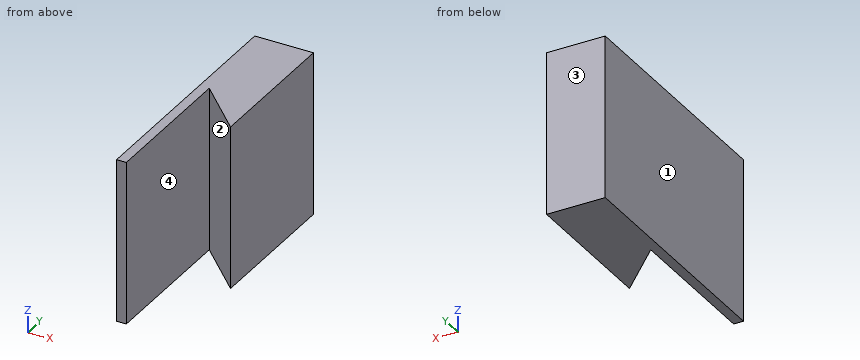
Autodesk Fusion 360 part; units mm, degrees
sketch "Sketch1" plane through (0, 0, 0) normal (0, 0, 1) x (1, 0, 0) in component "generic_holder"
  line L0 (0, 0) -> (-15, 15)
  line L1 (-15, 15) -> (-15, 45)
  line L2 (-15, 45) -> (0, 45)
  line L3 (0, 45) -> (0, 0)
  line L4 (-15, 45) -> (-18, 45)
  line L5 (-18, 45) -> (-18, -30)
  line L6 (-18, -30) -> (-15, -30)
  line L7 (-15, -30) -> (-15, 45)
  dimension "d2" = 15
  dimension "d3" = 30
  dimension "d4" = 75
  dimension "d5" = 3
  dimension "d9" = 45
extrude "Extrude1" add sketch "Sketch1" along normal blind 50 in component "generic_holder"
component "generic_holder" placed x (1, 0, 0) y (0, 1, 0) z (0, 0, 1) at (0, 0, 0)
equation "d2 = cleat_thickness"
equation "d3 = cleat_short_hight"
equation "d4 = front_plate_hight"
equation "d5 = cleat_front_plate_thickness"
equation "cleat_thickness = 15 mm"
equation "cleat_long_hight = 45 mm"
equation "cleat_short_hight = 30 mm"
equation "d9 = cleat_long_hight"
equation "cleat_front_plate_thickness = 3 mm"
equation "front_plate_hight = 75 mm"
equation "cleat_width = 50 mm"
equation "d13 = cleat_width"
Input: part model. Units: mm. Frame: model coordinates. Face numbers are marked on the shaded views. Give positions to 0.01 mm unless a question says otherwise; leave off trailing zeros. Loops run counter-clockwise (first coordinate to the right, second up) from the corner with the lowest first, then second, coordinate; pieces in that order, holes last. Notation, with made-up numbers: M -14.5,-38 L 3.5,-38 A17 cw 3.5,-12 Z; hole C 81,28.25 d3. An arc over 180 degrees is marked long. Use one line per item in the form item = value.
1. Line query: L1, parallel to X at y = 14, z = 26; L2, parallel to X at y = -11, z = 39; L3, parallel to Y at x = -9, z = 21.5. Output: solid intervals per line, ascending.
Numbers:
L1 = -18 to -15, -14 to 0
L2 = -18 to -15
L3 = 9 to 45
2. Section query C-C, the plane z = 43. Return the cut outline in (x, y).
Numbers:
outline = M -18,-30 L -15,-30 L -15,15 L 0,0 L 0,45 L -18,45 Z
3. Section query A-A, the plane y = 10.5. Return the cut outline in (x, z).
Numbers:
outline = M -18,0 L -15,0 L -15,50 L -18,50 Z; M -10.5,0 L 0,0 L 0,50 L -10.5,50 Z
4. Pull-direction query (X, two-part tool) for the marked faces 1, 2, 3 and 4; classes: released by +X, released by -X, zero draft, split by the parting line, or undercut.
Numbers:
face_1 = released by -X
face_2 = undercut
face_3 = zero draft
face_4 = undercut
5. Section query D-D, the plane y = -6. Return the cut outline in (x, z), and give its area (3 significant figures).
Numbers:
outline = M -18,0 L -15,0 L -15,50 L -18,50 Z
area = 150 mm²
6. Section query B-B, the plane x = -12.75. Return the cut outline in (y, z), and give its area (3 significant figures).
Numbers:
outline = M 12.75,0 L 45,0 L 45,50 L 12.75,50 Z
area = 1,610 mm²
